CAD build for the part. Positions are in the model's coordinates, mm. A direction names the side the tool comes from. Round coordinates to 2 decimals unless told otherwise and drop trailing zeros. Order: outer loops, then holes, each group sorted by start corner. A loop starts at its lowest first (then second) coordinate and runs counter-clockwise, first axis right, second up. Notation, with made-up numbers: (60.25, 28) - (90.25, 28) arc R15 cw to (90.25, 48) - close; hole circle Ø2 at (60, 51). An arc over 180 degrees is marked (long way). Write item = value, one per line.
from build123d import *

# Parameters (mm, degrees)
SKETCH1_W           = 15
SKETCH1_H           = 15.7
BOSS_EXTRUDE1_DEPTH = 0.8
BOSS_EXTRUDE2_DEPTH = 10.8


with BuildPart() as part:
    # Sketch1 → Boss-Extrude1 (new body)
    with BuildSketch(Plane(origin=(0, 0, 0), x_dir=(1, 0, 0), z_dir=(0, 1, 0))):
        with Locations((0.367290749, -0.172907489)):
            Rectangle(SKETCH1_W, SKETCH1_H)
    extrude(amount=BOSS_EXTRUDE1_DEPTH)

    # Sketch2 → Boss-Extrude2 (add)
    with BuildSketch(Plane.XY.offset(9.722907489)):
        with BuildLine():
            Line((-2.944438856, 2), (3.555561144, 2))
            ThreePointArc((3.555561144, 2), (5.155561144, 0.4), (3.555561144, -1.2))
            Line((3.555561144, -1.2), (-2.944438856, -1.2))
            ThreePointArc((-2.944438856, -1.2), (-4.544438856, 0.4), (-2.944438856, 2))
        make_face()
    extrude(amount=-BOSS_EXTRUDE2_DEPTH)


solid = part.part
(1) Tool access for faces 1 (the flat face through (0, -1, -1.077)), 2 (the flat face through (0, 0, -2)), 3 (the flat face through (0, 0.8, -2)), 4 (the flat face through (0, 1, -1.077)): list every direction of +Z, -Z, +X, -X, +Y, -Y with a clear straight run to the whole face (end or side of a thin tool).
Solved:
face_1 = -Z, +X, -X, -Y
face_2 = -Z, -Y
face_3 = -Z, +Y
face_4 = -Z, +X, -X, +Y
(2) Band-saw the part on C-C on y = 0.4. List the corners of the cut face in (x, z).
Solved:
outline = (-7.13, -7.68) - (7.87, -7.68) - (7.87, 8.02) - (5.16, 8.02) - (5.16, 9.72) - (-4.54, 9.72) - (-4.54, 8.02) - (-7.13, 8.02) - close
(3) Band-saw the part on D-D on x = 6. List the corners of the cut face in (y, z), plus the area to 3 significant figures.
Solved:
outline = (0, -7.68) - (0.8, -7.68) - (0.8, 8.02) - (0, 8.02) - close
area = 12.6 mm²
(4) Drop flat-ended pins along their axis: pin 1 (0.6 mm diameter, centred on x = 0, y = -0.5, fed in from -Z); pin 2 (0.6 mm diameter, centred on x = -5.5, y = 0.5, fed in from +Z). Give the stop position or say it passes through.
Solved:
pin_1 = -1.08
pin_2 = 8.02
(5) Band-saw the part on A-A on x = -1.25. List the corners of the cut face in (y, z).
Solved:
outline = (-1.2, -1.08) - (0, -1.08) - (0, -7.68) - (0.8, -7.68) - (0.8, -1.08) - (2, -1.08) - (2, 9.72) - (-1.2, 9.72) - close
(6) Probe line 1 along Z through (x, y) = (-2, 1.35); line 2 along Y through (x, z) = (6.75, 2.5); line 3 along Z through (x, y) = (-5.25, 0.4). List the from-to ranges inside material, lowest first.
Solved:
line_1 = -1.08 to 9.72
line_2 = 0 to 0.8
line_3 = -7.68 to 8.02
(7) Band-saw the part on B-B on z = 4. List the corners of the cut face in (x, y), plus the area to 3 significant figures.
Solved:
outline = (-7.13, 0) - (-4.49, 0) arc R1.6 ccw to (-2.94, -1.2) - (3.56, -1.2) arc R1.6 ccw to (5.1, 0) - (7.87, 0) - (7.87, 0.8) - (5.1, 0.8) arc R1.6 ccw to (3.56, 2) - (-2.94, 2) arc R1.6 ccw to (-4.49, 0.8) - (-7.13, 0.8) - close
area = 33.1 mm²
